Read the model definition and answer for the solid it produces. Units are mm, in the model's axes. Face numbers are marked on the shaded views. A direction names the side the tool comes from. Coordinates: 2 decimals unless noted, no trailing zeros. Write each loop counter-clockwise with the first axis right and the second up, starting at its lowest first coordinate (ties: lowest second). Pieces come first, ordered by that corner, then holes. Notation, with made-up numbers: (52, 80.25) -> (77, 80.25) arc R11 ccw to (77, 100.25) -> close; hole circle Ø11 at (-12, -17.5). An arc over 180 degrees is marked (long way). One line per item, written item: value. Start each with the question number.
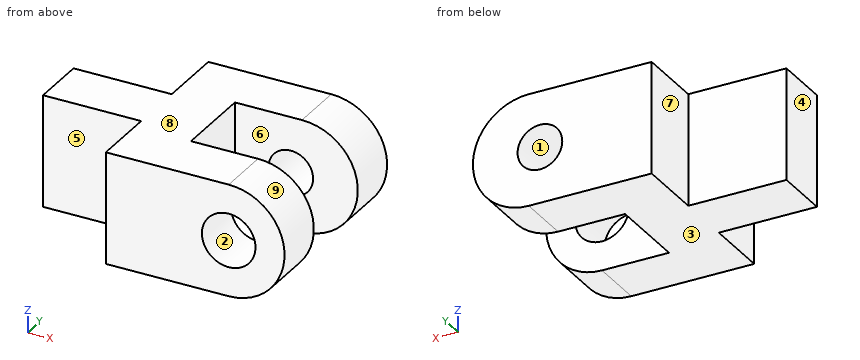
from build123d import *

# Parameters (mm, degrees)
BOSS_EXTRUDE1_DEPTH = 25
SKETCH2_R           = 12.5
BOSS_EXTRUDE2_DEPTH = 12
SKETCH3_R           = 12.5
BOSS_EXTRUDE3_DEPTH = 12
SKETCH4_R           = 5
CUT_EXTRUDE1_DEPTH  = 12
SKETCH5_R           = 6
CUT_EXTRUDE2_DEPTH  = 12


with BuildPart() as part:
    # Sketch1 → Boss-Extrude1 (new body)
    with BuildSketch(Plane.XY):
        Polygon((0, 0), (21.96969697, 0), (21.96969697, -14.5), (49.46969697, -14.5), (49.46969697, -2.5), (34.46969697, -2.5), (34.46969697, 15.5), (49.46969697, 15.5), (49.46969697, 27.5), (21.96969697, 27.5), (21.96969697, 12.5), (0, 12.5), align=None)
    extrude(amount=BOSS_EXTRUDE1_DEPTH)

    # Sketch2 → Boss-Extrude2 (add)
    with BuildSketch(Plane(origin=(0, 27.5, 0), x_dir=(1, 0, 0), z_dir=(0, 1, 0))):
        with Locations((49.46969697, -12.5)):
            Circle(SKETCH2_R)
    extrude(amount=-BOSS_EXTRUDE2_DEPTH)

    # Sketch3 → Boss-Extrude3 (add)
    with BuildSketch(Plane(origin=(0, -2.5, 0), x_dir=(1, 0, 0), z_dir=(0, 1, 0))):
        with Locations((49.46969697, -12.5)):
            Circle(SKETCH3_R)
    extrude(amount=-BOSS_EXTRUDE3_DEPTH)

    # Sketch4 → Cut-Extrude1 (cut)
    with BuildSketch(Plane(origin=(0, 27.5, 0), x_dir=(1, 0, 0), z_dir=(0, 1, 0))):
        with Locations(Location((46.96969697, -12.5, 0), (0, 0, 180))):
            Circle(SKETCH4_R)
    extrude(amount=-CUT_EXTRUDE1_DEPTH, mode=Mode.SUBTRACT)

    # Sketch5 → Cut-Extrude2 (cut)
    with BuildSketch(Plane(origin=(0, -2.5, 0), x_dir=(1, 0, 0), z_dir=(0, 1, 0))):
        with Locations(Location((49.46969697, -12.5, 0), (0, 0, 180))):
            Circle(SKETCH5_R)
    extrude(amount=-CUT_EXTRUDE2_DEPTH, mode=Mode.SUBTRACT)


solid = part.part
1. A cutting plane is placed at D-D on z = 12.5. Give the vertices of the cut face in (x, y).
2. For a pull along X with two mould halves and no side action, classify the marked faces 1, 2, 3 and 4 as +X half, -X half, draft (parallel to the pull), parting line (faces both ways), or undercut.
3. A cutting plane is placed at B-B on z = 9.5. Give the vertices of the cut face in (x, y).
4. A cutting plane is placed at A-A on y = -9. Give the vertices of the cut face in (x, z), then the cut area to 3 significant figures.
5. Given pin 1 (6.5 mm diameter, centred on x = 6.5, z = 13, fed in from -Y), flat-ended and moving along its own axis, determine where the tip first touches the part or whether it passes through.
6. Find the intervals of material crossed by probe 1 along Y at (x, z) = (42, 15.75); probe 2 along Y at (x, z) = (12, 7.5); probe 3 along X at (y, z) = (1, 9.25), in increasing order. Write a range as from..to.
7. A cutting plane is placed at C-C on y = 17. Give the vertices of the cut face in (x, z), then the cut area to 3 significant figures.
8. A tool of negligible diameter and unlimited length cuts with its end or side. For the marked faces 5, 6, 7, 8 and 9, from which of +Z, -Z, +X, -X, +Y, -Y can it reach the whole face along a straight path? Write none if from no direction.
Derived:
1. outline: (0, 0) -> (21.97, 0) -> (21.97, -14.5) -> (43.47, -14.5) -> (43.47, -2.5) -> (34.47, -2.5) -> (34.47, 15.5) -> (41.97, 15.5) -> (41.97, 27.5) -> (21.97, 27.5) -> (21.97, 12.5) -> (0, 12.5) -> close; (51.97, 15.5) -> (61.97, 15.5) -> (61.97, 27.5) -> (51.97, 27.5) -> close; (55.47, -14.5) -> (61.97, -14.5) -> (61.97, -2.5) -> (55.47, -2.5) -> close
2. face 1: undercut
2. face 2: undercut
2. face 3: draft
2. face 4: -X half
3. outline: (0, 0) -> (21.97, 0) -> (21.97, -14.5) -> (44.27, -14.5) -> (44.27, -2.5) -> (34.47, -2.5) -> (34.47, 15.5) -> (42.97, 15.5) -> (42.97, 27.5) -> (21.97, 27.5) -> (21.97, 12.5) -> (0, 12.5) -> close; (50.97, 15.5) -> (61.6, 15.5) -> (61.6, 27.5) -> (50.97, 27.5) -> close; (54.67, -14.5) -> (61.6, -14.5) -> (61.6, -2.5) -> (54.67, -2.5) -> close
4. outline: (21.97, 0) -> (49.47, 0) arc R12.5 ccw to (49.47, 25) -> (21.97, 25) -> close; hole circle Ø12 at (49.47, 12.5)
4. area: 820 mm2
5. pin 1: stops at y = 0
6. probe 1: y = -14.5..-2.5, 15.5..27.5
6. probe 2: y = 0..12.5
6. probe 3: x = 0..34.47
7. outline: (21.97, 0) -> (49.47, 0) arc R12.5 ccw to (49.47, 25) -> (21.97, 25) -> close; hole circle Ø10 at (46.97, 12.5)
7. area: 854 mm2
8. face 5: +Z, -Z, -X, -Y
8. face 6: +Z, -Z, +X
8. face 7: +Z, -Z, -X, +Y
8. face 8: +Z, +X, -X, +Y, -Y
8. face 9: +X, +Y, -Y
